For this review, use the dimensioned drawing (mm, ordinates from the lowest corner) and the shaded views. Give positions to 0.01 mm unless a question says otherwise; leave off trailing zeros. Order: outer loops, then holes, each group sorted by start corner. A loop starts at its lowest first (then second) coordinate and runs counter-clockwise, first axis right, second up. Notation, with made-up numbers: M 76,45.25 L 123,45.25 A27 cw 123,81.25 Z; hole C 38.5,49 d3. An arc over 180 degrees is marked long. One line per question, with ' | ' between items. Start each with the question number.
1. Wall thickness on L1, parallel to Y at x = 2, z = 24.5; L2, parallel to Y at x = 1.1, z = 28.5; L3, parallel to Y at x = 0.2, z = 5.5: over which ranges is each line inside the solid? List them lowest first.
2. We need section B-B on x = 0.8. Count the separate pieces of the cut face and the enclosed holes in it, then the cut area to 3 significant figures.
3. Insertion check: P1, Ø0.8, axis at x = 1.5, y = 53.5, coming from the -Z side; P2, Ø1.5, axis at x = 2, y = 7.5, coming from the -Z side; P3, Ø1.2, axis at x = 1.5, y = 54, coming from the -Z side. Each pin has a flat end and moves straight along its axis. Give the tip position at first contact, or say it passes through.
4. We need section A-A on y = 38.7. Write out the cut boundary in (x, z).
5. We need section C-C on y = 28.5. Write out the cut boundary in (x, z).
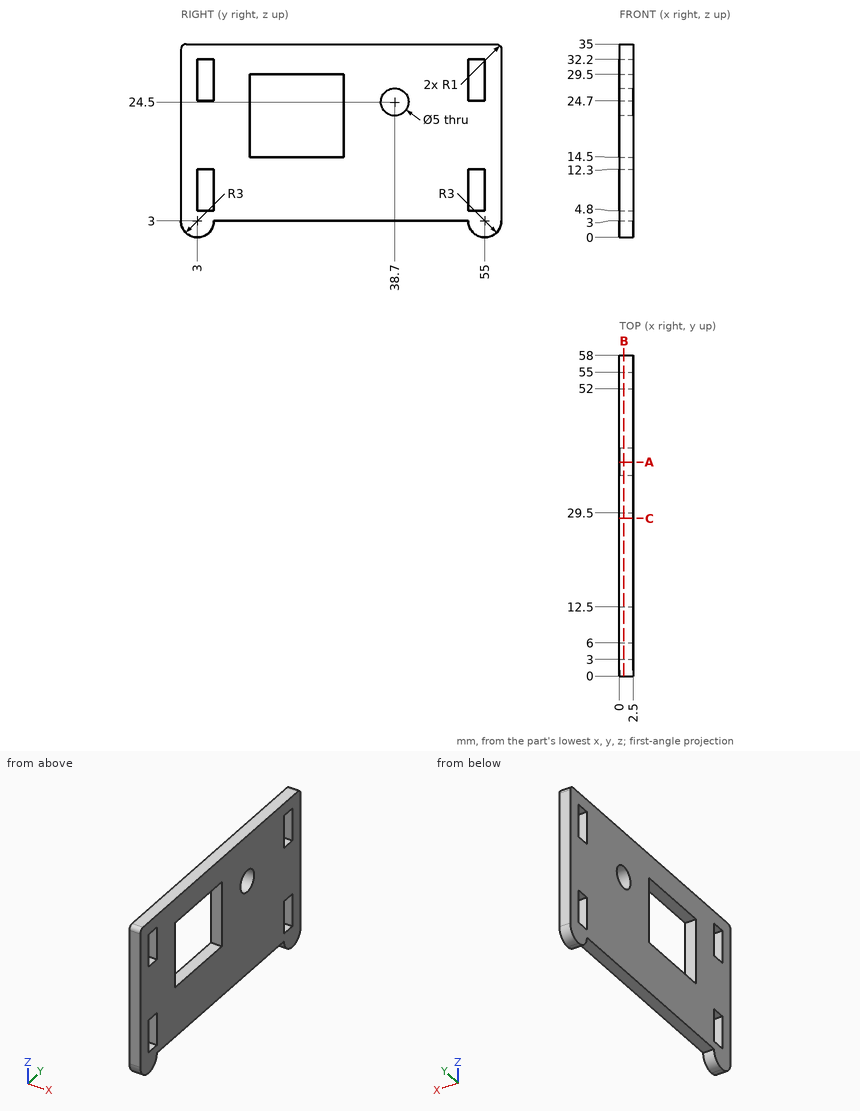
Entries:
1) L1: y = 0 to 12.5, 29.5 to 36.2, 41.2 to 58 | L2: y = 0 to 3, 6 to 12.5, 29.5 to 52, 55 to 58 | L3: y = 0 to 3, 6 to 52, 55 to 58
2) separate pieces: 1 | enclosed holes: 6 | area: 1,520 mm^2
3) P1: stops at z = 0.21 | P2: stops at z = 3 | P3: stops at z = 0.03
4) outline: M 0,3 L 2.5,3 L 2.5,22 L 0,22 Z; M 0,27 L 2.5,27 L 2.5,35 L 0,35 Z
5) outline: M 0,3 L 2.5,3 L 2.5,14.5 L 0,14.5 Z; M 0,29.5 L 2.5,29.5 L 2.5,35 L 0,35 Z
